Can you work these out from the model? Positions are in its coordinate system, mm. Face numbers are marked on the shaded views. A direction names the side the tool comes from. Coordinates: 2 decimals unless noted, no trailing zeros. Order: outer loops, then holes, each group sorted by start corner. A loop starts at its lowest first (then second) coordinate and runs counter-clockwise, first axis right, second up.
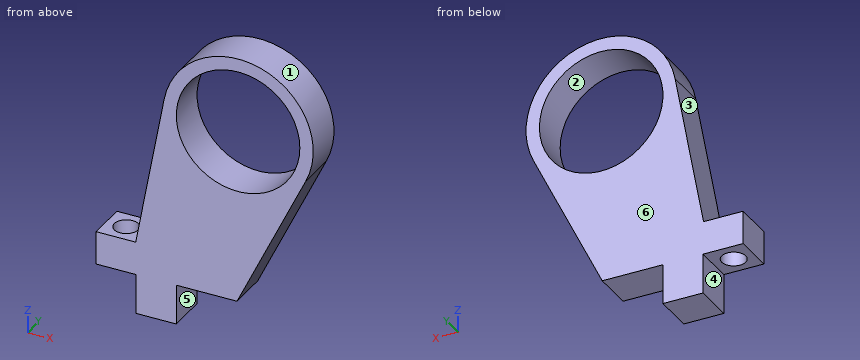
```python
from build123d import *

# Parameters (mm, degrees)
SKETCH1_R           = 9.25
BOSS_EXTRUDE1_DEPTH = 6
SKETCH2_R           = 1.8
CUT_EXTRUDE1_DEPTH  = 12


with BuildPart() as part:
    # Sketch1 → Boss-Extrude1 (new body)
    with BuildSketch(Plane(origin=(0, 0, 0), x_dir=(1, 0, 0), z_dir=(0, 1, 0))):
        with BuildLine():
            Line((-21.25, 26.25), (-15.25, 26.25))
            Line((-15.25, 26.25), (-15.25, 32.25))
            Line((-15.25, 32.25), (-9.25, 32.25))
            Line((-9.25, 32.25), (-9.25, 26.25))
            Line((-9.25, 26.25), (-0.158743734, 26.25))
            Line((-0.158743734, 26.25), (10.135163922, 4.882719763))
            ThreePointArc((10.135163922, 4.882719763), (3.485591088, -10.696408499), (-11.066060992, -2.026029152))
            Line((-11.066060992, -2.026029152), (-15.327551476, 21.25))
            Line((-15.327551476, 21.25), (-21.25, 21.25))
            Line((-21.25, 21.25), (-21.25, 26.25))
        make_face()
        Circle(SKETCH1_R, mode=Mode.SUBTRACT)
    extrude(amount=BOSS_EXTRUDE1_DEPTH)

    # Sketch2 → Cut-Extrude1 (cut, through all)
    with BuildSketch(Plane.XY.offset(-21.25)):
        with Locations((-18.288775738, 3)):
            Circle(SKETCH2_R)
    extrude(amount=-CUT_EXTRUDE1_DEPTH, mode=Mode.SUBTRACT)


solid = part.part
```
1. Imagine slicing it at B-B on x = 1.5. Please give me the cut outline in (y, z).
Completed:
outline: (0, -22.81) - (6, -22.81) - (6, -9.13) - (0, -9.13) - close; (0, 9.13) - (6, 9.13) - (6, 11.15) - (0, 11.15) - close
2. Imagine slicing it at C-C on z = 0. Please give me the cut outline in (x, y), then the cut area to 3 significant figures.
Completed:
outline: (-11.44, 0) - (-9.25, 0) - (-9.25, 6) - (-11.44, 6) - close; (9.25, 0) - (11.25, 0) - (11.25, 6) - (9.25, 6) - close
area: 25.1 mm2
3. Please list where these lines run through material, in increasing order: probe 1 along X at (y, z) = (5.4, -27); probe 2 along Z at (x, y) = (0, 4.65); probe 3 along Z at (x, y) = (6, 2.6).
Completed:
probe 1: x = -15.25 to -9.25
probe 2: z = -25.92 to -9.25, 9.25 to 11.25
probe 3: z = -13.47 to -7.04, 7.04 to 9.52
4. On a 3-axis mill with a long thin cutter (end or side, diameter ignored), from which of +Z, -Z, +X, -X, +Y, -Y can I reach the whole of each face in a straight line? I mean the marked faces 5 and 6. Say none if no direction works.
Completed:
face 5: -Z, +X, +Y, -Y
face 6: +Z, -Z, +X, -X, +Y
5. I'm going to push flat-ended pins straight in: pin 1 (1 mm diameter, centred on x = 4.5, y = 3.5, fed in from -Z); pin 2 (1 mm diameter, centred on y = 0.5, z = -1, fed in from +X); pin 3 (3 mm diameter, centred on x = -17.5, y = 4, fed in from -Z). Where does each tip first touch, or does it pass through?
Completed:
pin 1: stops at z = -17.62
pin 2: stops at x = 11.24
pin 3: stops at z = -26.25
6. Imagine slicing it at A-A on y = 3. Please give me the cut outline in (x, z), then the cut area to 3 significant figures.
Completed:
outline: (-21.25, -26.25) - (-20.09, -26.25) - (-20.09, -21.25) - (-21.25, -21.25) - close; (-16.49, -26.25) - (-15.25, -26.25) - (-15.25, -32.25) - (-9.25, -32.25) - (-9.25, -26.25) - (-0.16, -26.25) - (10.14, -4.88) arc R11.25 ccw (long way) to (-11.07, 2.03) - (-15.33, -21.25) - (-16.49, -21.25) - close; hole circle Ø18.5 at (0, 0)
area: 498 mm2
7. Thinking about a two-plate mould opening in Z: for the marked faces 1, 2, 3 and 4, which applies, pulls with the +Z half, pulls with the -Z half, needs draft (parallel to the pull), parting line crosses it, or undercut?
Completed:
face 1: parting line crosses it
face 2: undercut
face 3: pulls with the +Z half
face 4: needs draft
8. Imagine slicing it at D-D on z = -13. Please give me the cut outline in (x, y).
Completed:
outline: (-13.82, 0) - (6.22, 0) - (6.22, 6) - (-13.82, 6) - close
